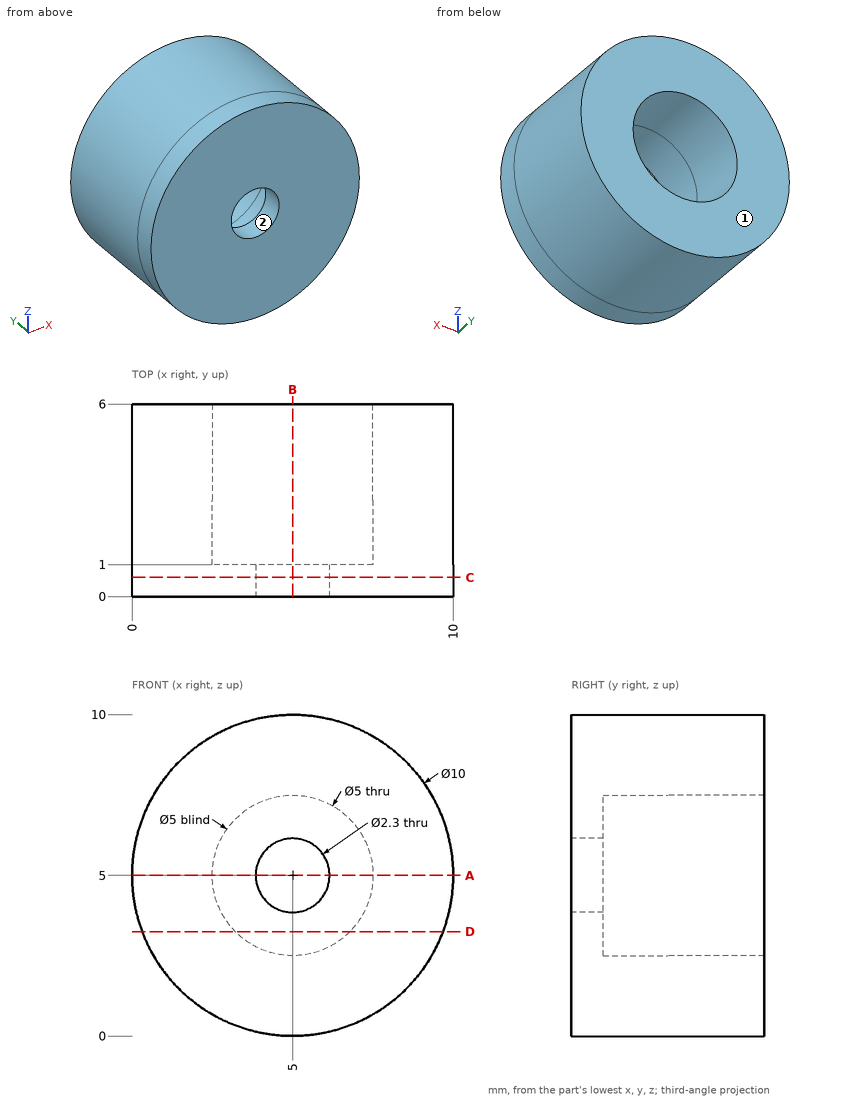
Part print with two shaded views. Sizes in mm from the minimum x, y, z corner. Coordinates: 2 decimals unless noted, no trailing zeros. Write each loop counter-clockwise with the first axis right and the second up, starting at its lowest first coordinate (ties: lowest second). Pieces come first, ordered by that corner, then holes. Notation, with made-up numbers: M 20,34 L 77,34 A13 ccw 77,52 Z; hole C 71,88 d10. An arc over 180 degrees is marked long. Return JSON: item names as keys, results as strings.
Item 1: Probe line 1 (X direction, y = 1.95, z = 5); line 2 (Y direction, x = 6.25, z = 4.5). List the from-to ranges inside material, lowest first. Write a range as from..to.
Findings below:
{"line 1": "x = 0..2.5, 7.5..10", "line 2": "y = 0..1"}
Item 2: Slice it at A-A, the plane z = 5. Write the cut outline in (x, y), and give its area (3 significant figures).
Findings below:
{"outline": "M 0,0 L 3.85,0 L 3.85,1 L 2.5,1 L 2.5,6 L 0,6 Z; M 6.15,0 L 10,0 L 10,6 L 7.5,6 L 7.5,1 L 6.15,1 Z", "area": "32.7 mm2"}
Item 3: Drop flat-ended pins along their axis: pin 1 Ø1.5 at (x, z) = (4.5, 4.5) entering from +Y; pin 2 Ø2 at (x, z) = (5, 5) entering from +Y (3 decimals). Give the stop position or say it passes through.
Findings below:
{"pin 1": "stops at y = 1", "pin 2": "passes through"}
Item 4: Slice it at D-D, the plane z = 3.25. Write the cut outline in (x, y), and give its area (3 significant figures).
Findings below:
{"outline": "M 0.32,0 L 9.68,0 L 9.68,6 L 6.79,6 L 6.79,1 L 3.21,1 L 3.21,6 L 0.32,6 Z", "area": "38.4 mm2"}
Item 5: Slice it at B-B, the plane x = 5. Write the cut outline in (y, z).
Findings below:
{"outline": "M 0,0 L 6,0 L 6,2.5 L 1,2.5 L 1,3.85 L 0,3.85 Z; M 0,6.15 L 1,6.15 L 1,7.5 L 6,7.5 L 6,10 L 0,10 Z"}
Item 6: Slice it at C-C, the plane y = 0.6. Write the cut outline in (x, z), and give its area (3 significant figures).
Findings below:
{"outline": "C 5,5 d10; hole C 5,5 d2.3", "area": "74.4 mm2"}
Item 7: Two-plate mould, pull along X, no slides. Class the marked faces 1 and 2: +X half, -X half, draft (parallel to the pull), parting line (faces both ways), or undercut.
Findings below:
{"face 1": "draft", "face 2": "undercut"}
